from build123d import *

# Parameters (mm, degrees)
SKETCH_4_R          = 1.5
CUT_EXTRUDE_1_DEPTH = 64.371918071


with BuildPart() as part:
    # 草图2 → 旋转1 (revolve)
    with BuildSketch(Plane.XY, mode=Mode.PRIVATE) as revolve_1_sk:
        Polygon((34, 12), (34, 0), (40, 0), (40, 10), (44, 10), (44, 12), align=None)
    revolve(revolve_1_sk.sketch.rotate(Axis((0, 0, 0), (0, 1, 0)), 90), axis=Axis((0, 0, 0), (0, 1, 0)))

    # 草图4 → 切除-拉伸1 (cut, through all)
    with BuildSketch(Plane(origin=(0, 0, 0), x_dir=(1, 0, 0), z_dir=(0, 1, 0))):
        with Locations(Location((0, 37, 0), (0, 0, 270))):
            Circle(SKETCH_4_R)
        with Locations(Location((32.04293994, 18.5, 0), (0, 0, 270))):
            Circle(SKETCH_4_R)
        with Locations(Location((32.04293994, -18.5, 0), (0, 0, 270))):
            Circle(SKETCH_4_R)
        with Locations(Location((0, -37, 0), (0, 0, 270))):
            Circle(SKETCH_4_R)
        with Locations(Location((-32.04293994, -18.5, 0), (0, 0, 270))):
            Circle(SKETCH_4_R)
        with Locations(Location((-32.04293994, 18.5, 0), (0, 0, 270))):
            Circle(SKETCH_4_R)
    extrude(amount=CUT_EXTRUDE_1_DEPTH, mode=Mode.SUBTRACT)


solid = part.part
Design review of the part built by this model. Coordinates are the model's own, in mm. A direction names the side the tool comes from. Give positions to 0.01 mm unless a question says otherwise; leave off trailing zeros. Loops run counter-clockwise (first coordinate to the right, second up) from the corner with the lowest first, then second, coordinate; pieces in that order, holes last. Notation, with made-up numbers: M -32,-17.5 L -2,-17.5 A14 cw -2,1.5 Z; hole C 57.25,16.25 d5. An arc over 180 degrees is marked long. Answer as a JSON object with one key per item and string values.
Item 1: We need section C-C (z = 29). State the section outline as (x, y) points, and give its area (3 significant figures).
Output values:
{"outline": "M -33.09,10 L -27.55,10 L -27.55,0 L -17.75,0 L -17.75,12 L -33.09,12 Z; M 17.75,0 L 27.55,0 L 27.55,10 L 33.09,10 L 33.09,12 L 17.75,12 Z", "area": "257 mm2"}
Item 2: Wall thickness on line 1 along X through (y, z) = (3, -0.5); line 2 along X through (y, z) = (3.75, -18.5); line 3 along X through (y, z) = (8.75, 18): over which ranges is each line inside the solid? List them lowest first.
Output values:
{"line 1": "x = -40 to -34, 34 to 40", "line 2": "x = -35.46 to -33.54, -30.54 to -28.53, 28.53 to 30.54, 33.54 to 35.46", "line 3": "x = -35.72 to -33.46, -30.63 to -28.84, 28.84 to 30.63, 33.46 to 35.72"}
Item 3: For P1, Ø6, axis at y = 9, z = 8.5, coming from the -X side; P2, Ø3, axis at y = 5.5, z = -28.5, coming from the -X side; P3, Ø1.5, axis at x = 8.5, y = 5.5, coming from the -Z side, all flat-tipped, find the tip position at first contact; note any pin that passes through.
Output values:
{"P1": "stops at x = -43.63", "P2": "stops at x = -29.51", "P3": "stops at z = -39.24"}
Item 4: Machinability: for faces 5 (the face through (-1.76, 5.07, 39.96)), 6 (the face through (-32, 6, -20)), which of the approach directions +Z, -Z, +X, -X, +Y, -Y give a long, thin tool a straight path to every point of the face, cutting with its end or side? Answer none if there is none.
Output values:
{"face 5": "-Y", "face 6": "+Y, -Y"}
Item 5: Mouldability with a two-part tool opening along X and no side actions: class faces 1 (the face through (-0.9, 5.9, -38.2)), 2 (the face through (32, 6, 17)), 3 (the face through (29.4, 0, -18)), 4 (the face through (42.954, 11.014, 9.538)) as pulls with the +X half, pulls with the -X half, needs draft (parallel to the pull), parting line crosses it, or undercut.
Output values:
{"face 1": "undercut", "face 2": "undercut", "face 3": "needs draft", "face 4": "parting line crosses it"}
Item 6: We need section A-A (x = 0). State the section outline as (y, z) points.
Output values:
{"outline": "M 0,-40 L 10,-40 L 10,-44 L 12,-44 L 12,-38.5 L 0,-38.5 Z; M 0,-35.5 L 12,-35.5 L 12,-34 L 0,-34 Z; M 0,34 L 12,34 L 12,35.5 L 0,35.5 Z; M 0,38.5 L 12,38.5 L 12,44 L 10,44 L 10,40 L 0,40 Z"}
Item 7: We need section B-B (z = -18.5). State the section outline as (x, y) points.
Output values:
{"outline": "M -39.92,10 L -35.46,10 L -35.46,0 L -33.54,0 L -33.54,12 L -39.92,12 Z; M -30.54,0 L -28.53,0 L -28.53,12 L -30.54,12 Z; M 28.53,0 L 30.54,0 L 30.54,12 L 28.53,12 Z; M 33.54,0 L 35.46,0 L 35.46,10 L 39.92,10 L 39.92,12 L 33.54,12 Z"}
Item 8: We need section D-D (x = -10.5). State the section outline as (y, z) points.
Output values:
{"outline": "M 0,-38.6 L 10,-38.6 L 10,-42.73 L 12,-42.73 L 12,-32.34 L 0,-32.34 Z; M 0,32.34 L 12,32.34 L 12,42.73 L 10,42.73 L 10,38.6 L 0,38.6 Z"}
